Geometry: final body of the model. Coordinates: model frame, mm. A direction names the side the tool comes from. Coordinates: 2 decimals unless noted, no trailing zeros. Order: outer loops, then holes, each group sorted by start corner. A loop starts at its lowest first (then second) coordinate and runs counter-clockwise, first axis right, second up. Notation, with made-up numbers: M 32,47 L 36,47 A20 ccw 36,59 Z; hole C 75,59.25 d5. An arc over 180 degrees is marked long. Write item = value, one per line.
from build123d import *

# Parameters (mm, degrees)
BOSS_EXTRUDE1_DEPTH = 20
SKETCH2_W           = 5
SKETCH2_H           = 3
BOSS_EXTRUDE2_DEPTH = 120


with BuildPart() as part:
    # Sketch1 → Boss-Extrude1 (new body)
    with BuildSketch(Plane.XY):
        with BuildLine():
            Line((-24.05, 64.8), (-24.05, 41.8))
            Line((-24.05, 41.8), (24.05, 41.8))
            Line((24.05, 41.8), (24.05, 64.8))
            add(Edge.make_bspline(
                [(24.05, 64.8), (22.187774265, 77.400108054), (20.594686421, 64.8)],
                knots=[0, 0, 0, 1, 1, 1], degree=2))
            Line((20.594686421, 64.8), (20.594686421, 44.8))
            Line((20.594686421, 44.8), (-20.594686421, 44.8))
            Line((-20.594686421, 44.8), (-20.594686421, 64.8))
            add(Edge.make_bspline(
                [(-24.05, 64.8), (-22.187774265, 77.400108054), (-20.594686421, 64.8)],
                knots=[0, 0, 0, 1, 1, 1], degree=2))
        make_face()
    extrude(amount=BOSS_EXTRUDE1_DEPTH)

    # Sketch2 → Boss-Extrude2 (add)
    with BuildSketch(Plane.XY.offset(20)):
        with Locations((-26.55, 43.3)):
            Rectangle(SKETCH2_W, SKETCH2_H)
        Polygon((-24.05, 44.8), (-24.05, 41.8), (24.05, 41.8), (24.05, 44.8), (20.594686421, 44.8), (-20.594686421, 44.8), align=None)
        with Locations((26.55, 43.3)):
            Rectangle(SKETCH2_W, SKETCH2_H)
    extrude(amount=BOSS_EXTRUDE2_DEPTH)


solid = part.part
1) Section A-A, the plane y = 54.25. Return loops of the section in (x, z), and give its area (3 significant figures).
Numbers:
outline = M -24.05,0 L -20.59,0 L -20.59,20 L -24.05,20 Z; M 20.59,0 L 24.05,0 L 24.05,20 L 20.59,20 Z
area = 138 mm²
2) Line query: L1, parallel to X at y = 57.75, z = 11.5; L2, parallel to Y at x = -24, z = 86.5; L3, parallel to Z at x = 21.5, y = 68.25. Output: solid intervals per line, ascending.
Numbers:
L1 = -24.05 to -20.59, 20.59 to 24.05
L2 = 41.8 to 44.8
L3 = 0 to 20
3) Set-up query: faces 4 (the face through (27, 43, 20)), 5 (the face through (-20.595, 55, 10)), 6 (the face through (22, 58, 20)). Return all of +Z, -Z, +X, -X, +Y, -Y with unobstructed straight access to the full face (end or side cutting, diameter ignored); none if empty.
Numbers:
face_4 = -Z, +X, +Y, -Y
face_5 = +Z, -Z, +Y
face_6 = +Z, +X, -X, +Y
4) Mould query, pull axis X, two halves, no side actions, for faces 1 (the face through (0, 44, 0)), 2 (the face through (29.05, 43, 79)), 3 (the face through (20.595, 55, 10)). Classes: pulls with the +X half, pulls with the -X half, needs draft (parallel to the pull), parting line crosses it, or undercut.
Numbers:
face_1 = needs draft
face_2 = pulls with the +X half
face_3 = undercut
5) Pin query (flat end, axial travel): pin 1 (3.5 mm diameter, centred on x = 25.5, y = 43, fed in from -Z); pin 2 (10 mm diameter, centred on y = 54.5, z = 14, fed in from -X); pin 3 (6 mm diameter, centred on y = 58.5, z = 8.5, fed in from +X); pin 4 (4 mm diameter, centred on x = -1.5, z = 113.5, fed in from +Y). Return the tip coordinate at first contact, or that it passes through.
Numbers:
pin_1 = 0
pin_2 = -24.05
pin_3 = 24.05
pin_4 = 44.8
6) Section B-B, the plane z = 27. Return loops of the section in (x, y).
Numbers:
outline = M -29.05,41.8 L 29.05,41.8 L 29.05,44.8 L -29.05,44.8 Z
7) Section C-C, the plane x = -12. Return loops of the section in (y, z).
Numbers:
outline = M 41.8,0 L 44.8,0 L 44.8,140 L 41.8,140 Z
